Source: CAD feature listing. Evaluate the final solid. Frame: model axes, mm. A direction names the side the tool comes from. Give positions to 0.01 mm unless a question says otherwise; leave off trailing zeros. Write each loop counter-clockwise with the first axis right and the second up, starting at its lowest first coordinate (ties: lowest second). Pieces come first, ordered by that corner, then holes.
```python
from build123d import *

# Parameters (mm, degrees)
SKETCH1_R           = 21
SKETCH1_R_2         = 15
BOSS_EXTRUDE1_DEPTH = 7
SKETCH2_R           = 19.73
SKETCH2_R_2         = 16.27
CUT_EXTRUDE1_DEPTH  = 0.254


with BuildPart() as part:
    # Sketch1 → Boss-Extrude1 (new body)
    with BuildSketch(Plane(origin=(0, 0, 0), x_dir=(1, 0, 0), z_dir=(0, 1, 0))):
        with Locations(Location((0, 0, 0), (0, 0, 270))):
            Circle(SKETCH1_R)
        with Locations(Location((0, 0, 0), (0, 0, 270))):
            Circle(SKETCH1_R_2, mode=Mode.SUBTRACT)
    extrude(amount=BOSS_EXTRUDE1_DEPTH)

    # Sketch2 → Cut-Extrude1 (cut)
    with BuildSketch(Plane(origin=(0, 7, 0), x_dir=(1, 0, 0), z_dir=(0, 1, 0))):
        with Locations(Location((0, 0, 0), (0, 0, 270))):
            Circle(SKETCH2_R)
        with Locations(Location((0, 0, 0), (0, 0, 270))):
            Circle(SKETCH2_R_2, mode=Mode.SUBTRACT)
    cut_extrude1 = extrude(amount=-CUT_EXTRUDE1_DEPTH, mode=Mode.SUBTRACT)

    # Mirror1: Cut-Extrude1 across plane
    add(cut_extrude1.mirror(Plane(origin=(0, 3.5, 0), x_dir=(0, 0, 1), z_dir=(0, -1, 0))), mode=Mode.SUBTRACT)


solid = part.part
```
1. Line query: L1, parallel to X at y = 0.2, z = 0; L2, parallel to X at y = 3, z = 0; L3, parallel to Y at x = 12, z = -15. Output: solid intervals per line, ascending.
2. Cut plane C-C, the plane y = 3.25. Return the cut outline in (x, z).
3. Contact query for flat-ended pins moving along their axis: P1, Ø1, axis at y = 2.5, z = -7.5, coming from the +X side; P2, Ø1.5, axis at x = 6, y = 6, coming from the -Z side. Output: stop coordinate, or through.
4. Cut plane B-B, the plane z = 0. Return the cut outline in (x, y), then the cut area to 3 significant figures.
5. Mould query, pull axis X, two halves, no side actions, for faces 3 (the flat face through (-14.39, 0, 4.74)), 4 (the flat face through (16.2, 0.254, 2.8)), 5 (the cylindrical face through (6.31, 3.45, 20.03)). Classes: +X half, -X half, draft (parallel to the pull), parting line (faces both ways), or undercut.
6. Access query for faces 1 (the cylindrical face through (0.66, 3.451, -14.985)), 2 (the flat face through (16.2, 6.746, 2.8)). Directions: +Z, -Z, +X, -X, +Y, -Y. A direction counts if a zero-diameter tool reaches every point of the face in a straight line with its end or side. Return the directions, or none.
7. Cut plane A-A, the plane x = 0. Return the cut outline in (y, z).
Response values:
1. L1: x = -21 to -19.73, -16.27 to -15, 15 to 16.27, 19.73 to 21
1. L2: x = -21 to -15, 15 to 21
1. L3: y = 0.25 to 6.75
2. outline: circle Ø42 at (0, 0); hole circle Ø30 at (0, 0)
3. P1: stops at x = 19.8
3. P2: stops at z = -20.33
4. outline: (-21, 0) - (-19.73, 0) - (-19.73, 0.25) - (-16.27, 0.25) - (-16.27, 0) - (-15, 0) - (-15, 7) - (-16.27, 7) - (-16.27, 6.75) - (-19.73, 6.75) - (-19.73, 7) - (-21, 7) - close; (15, 0) - (16.27, 0) - (16.27, 0.25) - (19.73, 0.25) - (19.73, 0) - (21, 0) - (21, 7) - (19.73, 7) - (19.73, 6.75) - (16.27, 6.75) - (16.27, 7) - (15, 7) - close
4. area: 80.5 mm2
5. face 3: draft
5. face 4: undercut
5. face 5: parting line
6. face 1: +Y, -Y
6. face 2: +Y
7. outline: (0, -21) - (7, -21) - (7, -19.73) - (6.75, -19.73) - (6.75, -16.27) - (7, -16.27) - (7, -15) - (0, -15) - (0, -16.27) - (0.25, -16.27) - (0.25, -19.73) - (0, -19.73) - close; (0, 15) - (7, 15) - (7, 16.27) - (6.75, 16.27) - (6.75, 19.73) - (7, 19.73) - (7, 21) - (0, 21) - (0, 19.73) - (0.25, 19.73) - (0.25, 16.27) - (0, 16.27) - close
